Geometry check sheet. Reference: the model listing, model coordinates, mm. A direction names the side the tool comes from. Coordinates: 2 decimals unless noted, no trailing zeros. Write each loop counter-clockwise with the first axis right and the second up, starting at its lowest first coordinate (ties: lowest second). Pieces come first, ordered by that corner, then holes. Notation, with made-up numbers: (-0.5, -20.5) -> (53.5, -20.5) arc R5 cw to (53.5, -14.5) -> close; hole circle Ø10 at (12.5, 21.25). An arc over 180 degrees is marked (long way). Use a Markdown table: item, result.
```python
from build123d import *

# Parameters (mm, degrees)
SKETCH1_W           = 55
SKETCH1_H           = 11
BOSS_EXTRUDE1_DEPTH = 35
CUT_EXTRUDE1_DEPTH  = 71
FILLET1_R           = 1
CUT_EXTRUDE2_DEPTH  = 71
CUT_EXTRUDE3_DEPTH  = 71
CUT_EXTRUDE4_DEPTH  = 7
FILLET2_R           = 0.5
SKETCH6_R           = 2.5527
CUT_EXTRUDE5_DEPTH  = 5


with BuildPart() as part:
    # Sketch1 → Boss-Extrude1 (new body, symmetric)
    with BuildSketch(Plane.XY):
        Rectangle(SKETCH1_W, SKETCH1_H)
    extrude(amount=BOSS_EXTRUDE1_DEPTH, both=True)

    # Sketch2 → Cut-Extrude1 (cut, through all)
    with BuildSketch(Plane.XY.offset(35)):
        with BuildLine():
            Line((-27.5, -0.5), (-16, -0.5))
            Line((-16, -0.5), (-16, -0.75))
            Line((-16, -0.75), (-18.95187639, -4.267909293))
            ThreePointArc((-18.95187639, -4.267909293), (-19.057073898, -5.066963696), (-18.377343058, -5.5))
            Line((-18.377343058, -5.5), (-27.5, -5.5))
            Line((-27.5, -5.5), (-27.5, -0.5))
        make_face()
    cut_extrude1 = extrude(amount=-CUT_EXTRUDE1_DEPTH, mode=Mode.SUBTRACT)

    # Mirror1: Cut-Extrude1 across plane
    add(cut_extrude1.mirror(Plane(origin=(0, 0, 0), x_dir=(0, 0, 1), z_dir=(1, 0, 0))), mode=Mode.SUBTRACT)

    # Fillet1
    fillet1_edges = [part.edges().sort_by_distance(p)[0] for p in [
        (-27.5, -0.5, 0),
        (27.5, -0.5, 0),
        (-27.5, 5.5, 0),
        (27.5, 5.5, 0),
    ]]
    fillet(fillet1_edges, radius=FILLET1_R)

    # Sketch3 → Cut-Extrude2 (cut, through all)
    with BuildSketch(Plane.XY.offset(35)):
        Polygon((-12.5, 5.5), (0, 5.5), (0, 5), (-12, 5), align=None)
    cut_extrude2 = extrude(amount=-CUT_EXTRUDE2_DEPTH, mode=Mode.SUBTRACT)

    # Mirror2: Cut-Extrude2 across plane
    add(cut_extrude2.mirror(Plane(origin=(0, 0, 0), x_dir=(0, 0, 1), z_dir=(1, 0, 0))), mode=Mode.SUBTRACT)

    # Sketch4 → Cut-Extrude3 (cut, through all)
    with BuildSketch(Plane.XY.offset(35)):
        with BuildLine():
            Line((-11, 1.5), (11, 1.5))
            Line((11, 1.5), (11, -1.5))
            ThreePointArc((11, -1.5), (10.853553391, -1.853553391), (10.5, -2))
            Line((10.5, -2), (-10.5, -2))
            ThreePointArc((-10.5, -2), (-10.853553391, -1.853553391), (-11, -1.5))
            Line((-11, -1.5), (-11, 1.5))
        make_face()
    extrude(amount=-CUT_EXTRUDE3_DEPTH, mode=Mode.SUBTRACT)

    # Sketch5 → Cut-Extrude4 (cut)
    with BuildSketch(Plane.XZ.offset(5.5)):
        with BuildLine():
            Line((-8, 28.5), (8, 28.5))
            ThreePointArc((8, 28.5), (10.121320344, 27.621320344), (11, 25.5))
            Line((11, 25.5), (11, -25.5))
            ThreePointArc((11, -25.5), (10.121320344, -27.621320344), (8, -28.5))
            Line((8, -28.5), (-8, -28.5))
            ThreePointArc((-8, -28.5), (-10.121320344, -27.621320344), (-11, -25.5))
            Line((-11, -25.5), (-11, 25.5))
            ThreePointArc((-11, 25.5), (-10.121320344, 27.621320344), (-8, 28.5))
        make_face()
    extrude(amount=-CUT_EXTRUDE4_DEPTH, mode=Mode.SUBTRACT)

    # Fillet2
    fillet2_edges = [part.edges().sort_by_distance(p)[0] for p in [
        (-11, 1.5, 0),
        (11, 1.5, 0),
    ]]
    fillet(fillet2_edges, radius=FILLET2_R)

    # Sketch6 → Cut-Extrude5 (cut, through all)
    with BuildSketch(Plane.XZ.offset(-1.5)):
        Circle(SKETCH6_R)
    extrude(amount=-CUT_EXTRUDE5_DEPTH, mode=Mode.SUBTRACT)


solid = part.part
```
Item 1: Section check B-B on x = 0. Record the boundary of the cut face in (y, z), then the cut area to 3 significant figures.
Answer block:
| item | result |
|---|---|
| outline | (-5.5, -35) -> (-2, -35) -> (-2, -28.5) -> (-5.5, -28.5) -> close; (-5.5, 28.5) -> (-2, 28.5) -> (-2, 35) -> (-5.5, 35) -> close; (1.5, -35) -> (5, -35) -> (5, -2.55) -> (1.5, -2.55) -> close; (1.5, 2.55) -> (5, 2.55) -> (5, 35) -> (1.5, 35) -> close |
| area | 273 mm^2 |
Item 2: Thickness scan on L1, parallel to Z at x = 0, y = 3.9; L2, parallel to Y at x = 8.5, z = 31; L3, parallel to Y at x = 22.5, z = -14. Record the ranges inside material, lowest first. Write a range as [from, to].
Answer block:
| item | result |
|---|---|
| L1 | z = [-35, -2.55], [2.55, 35] |
| L2 | y = [-5.5, -2], [1.5, 5] |
| L3 | y = [-0.5, 5.5] |
Item 3: Section check D-D on x = 23. Record the boundary of the cut face in (y, z), then the cut area to 3 significant figures.
Answer block:
| item | result |
|---|---|
| outline | (-0.5, -35) -> (5.5, -35) -> (5.5, 35) -> (-0.5, 35) -> close |
| area | 420 mm^2 |
Item 4: Depth check by flat-ended pin: P1, Ø4, axis at x = -6.5, z = 0.5, coming from the -Y side; P2, Ø2, axis at x = 8.5, z = 15.5, coming from the +Y side; P3, Ø3, axis at y = -4, z = 14.5, coming from the +X side; P4, Ø3, axis at x = 0, z = 0, coming from the +Y side. Enter the tip coordinate at first touch or a pass-through.
Answer block:
| item | result |
|---|---|
| P1 | stops at y = 1.5 |
| P2 | stops at y = 5 |
| P3 | stops at x = 19.13 |
| P4 | passes through |
Item 5: Tool access check on faces 1 (the cylindrical face through (-10.1, -3.53, -27.64)), 2 (the flat face through (-17.455, -2.484, 0.49)), 3 (the flat face through (21, -0.5, 0)). Record the directions out of +Z, -Z, +X, -X, +Y, -Y that give a thin tool (end or side, any length) a straight path to the whole face; none if there is none.
Answer block:
| item | result |
|---|---|
| face 1 | -Y |
| face 2 | +Z, -Z, -X |
| face 3 | +Z, -Z, +X |
Item 6: Section check C-C on z = 18.5. Record the boundary of the cut face in (x, y), then the cut area to 3 significant figures.
Answer block:
| item | result |
|---|---|
| outline | (-27.5, 0.5) arc R1 ccw to (-26.5, -0.5) -> (-16, -0.5) -> (-16, -0.75) -> (-18.95, -4.27) arc R0.75 ccw to (-18.38, -5.5) -> (-11, -5.5) -> (-11, 1) arc R0.5 cw to (-10.5, 1.5) -> (10.5, 1.5) arc R0.5 cw to (11, 1) -> (11, -5.5) -> (18.38, -5.5) arc R0.75 ccw to (18.95, -4.27) -> (16, -0.75) -> (16, -0.5) -> (26.5, -0.5) arc R1 ccw to (27.5, 0.5) -> (27.5, 4.5) arc R1 ccw to (26.5, 5.5) -> (12.5, 5.5) -> (12, 5) -> (-12, 5) -> (-12.5, 5.5) -> (-26.5, 5.5) arc R1 ccw to (-27.5, 4.5) -> close |
| area | 341 mm^2 |
Item 7: Mould release check, pull along Y, two halves, no side actions. Record for faces 4 (the flat face through (3, 5, 0)), 5 (the flat face through (17.455, -2.484, 0.49)), 6 (the flat face through (27.5, 2, 0)): +Y half, -Y half, draft (parallel to the pull), parting line (faces both ways), or undercut.
Answer block:
| item | result |
|---|---|
| face 4 | +Y half |
| face 5 | undercut |
| face 6 | draft |
